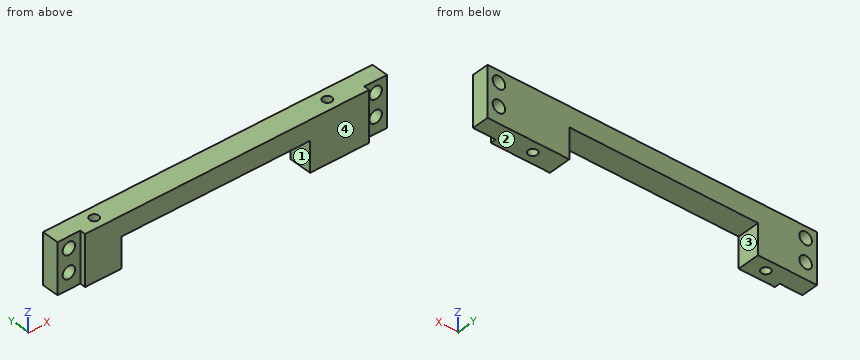
from build123d import *

# Parameters (mm, degrees)
MAIN_STOCK_START                         = 2.248090434
SKETCH_1_W                               = 57.95
SKETCH_1_H                               = 4
MAIN_STOCK_DEPTH                         = 8.851909566
SKETCH_2_W                               = 4
SKETCH_2_H                               = 1
CORNER_LEFT_RECTANGULAR_NOTCH_4X1_DEPTH  = 8.851909566
SKETCH_3_W                               = 4
SKETCH_3_H                               = 1
CORNER_RIGHT_RECTANGULAR_NOTCH_4X1_DEPTH = 8.851909566
SKETCH_4_R                               = 0.8
FRAME_2XD1P6_THROUGH_DEPTH               = 72.016485431
SKETCH_5_W                               = 33.203
SKETCH_5_H                               = 6.7
MERGED_INTERFACE_WINDOW_33P203X6P7_DEPTH = 4
SKETCH_6_R                               = 1.1
CORNER_REAR_4XD2P2_THROUGH_DEPTH         = 55.932071689


with BuildPart() as part:
    # 草图1 → Main_Stock (new body)
    with BuildSketch(Plane.XY.offset(MAIN_STOCK_START)):
        with Locations((24.675, 43.68)):
            Rectangle(SKETCH_1_W, SKETCH_1_H)
    extrude(amount=MAIN_STOCK_DEPTH)

    # 草图2 → Corner_Left_Rectangular_Notch_4x1 (cut)
    with BuildSketch(Plane.XY.offset(11.1)):
        with Locations((-2.3, 42.18)):
            Rectangle(SKETCH_2_W, SKETCH_2_H)
    extrude(amount=-CORNER_LEFT_RECTANGULAR_NOTCH_4X1_DEPTH, mode=Mode.SUBTRACT)

    # 草图3 → Corner_Right_Rectangular_Notch_4x1 (cut)
    with BuildSketch(Plane.XY.offset(11.1)):
        with Locations((51.65, 42.18)):
            Rectangle(SKETCH_3_W, SKETCH_3_H)
    extrude(amount=-CORNER_RIGHT_RECTANGULAR_NOTCH_4X1_DEPTH, mode=Mode.SUBTRACT)

    # 草图4 → Frame_2xD1p6_Through (cut, through all)
    with BuildSketch(Plane.XY.offset(11.1)):
        with Locations((3, 43.68)):
            Circle(SKETCH_4_R)
        with Locations((44, 43.68)):
            Circle(SKETCH_4_R)
    extrude(amount=-FRAME_2XD1P6_THROUGH_DEPTH, mode=Mode.SUBTRACT)

    # 草图5 → Merged_Interface_Window_33p203x6p7 (cut)
    with BuildSketch(Plane(origin=(0, 45.68, 0), x_dir=(1, 0, 0), z_dir=(0, 1, 0))):
        with Locations((22.6715, -4.25)):
            Rectangle(SKETCH_5_W, SKETCH_5_H)
    extrude(amount=-MERGED_INTERFACE_WINDOW_33P203X6P7_DEPTH, mode=Mode.SUBTRACT)

    # 草图6 → Corner_Rear_4xD2p2_Through (cut, through all)
    with BuildSketch(Plane(origin=(0, 45.68, 0), x_dir=(1, 0, 0), z_dir=(0, 1, 0))):
        with Locations(Location((-2.3, -5.1, 0), (0, 0, 270))):
            Circle(SKETCH_6_R)
        with Locations(Location((-2.3, -9.1, 0), (0, 0, 270))):
            Circle(SKETCH_6_R)
        with Locations(Location((51.65, -5.1, 0), (0, 0, 270))):
            Circle(SKETCH_6_R)
        with Locations(Location((51.65, -9.1, 0), (0, 0, 270))):
            Circle(SKETCH_6_R)
    extrude(amount=-CORNER_REAR_4XD2P2_THROUGH_DEPTH, mode=Mode.SUBTRACT)


solid = part.part
The model under review builds one solid part; all positions refer to its coordinate system, in mm. Face numbers are marked on the shaded views. A direction names the side the tool comes from. Coordinates: 2 decimals unless noted, no trailing zeros. Write each loop counter-clockwise with the first axis right and the second up, starting at its lowest first coordinate (ties: lowest second). Pieces come first, ordered by that corner, then holes. Notation, with made-up numbers: (25.25, 50.25) - (53.25, 50.25) arc R14 ccw to (53.25, 76.25) - close; hole circle Ø3 at (58, 67.5). An arc over 180 degrees is marked (long way). Answer as a JSON object with one key per item and string values. Group by question number.
1. Add section C-C (z = 9.1). Give the boundary of the cut face in (x, y), plus the area to 3 significant figures.
2. Mouldability with a two-part tool opening along X and no side actions: class the marked faces 3 and 4 as pulls with the +X half, pulls with the -X half, needs draft (parallel to the pull), parting line crosses it, or undercut.
3. Machinability: for the marked faces 1 and 2, which of the approach directions +Z, -Z, +X, -X, +Y, -Y give a long, thin tool a straight path to every point of the face, cutting with its end or side? Answer none if there is none.
4. Add section B-B (x = -2.3). Give the boundary of the cut face in (y, z).
5. Add section D-D (x = 44). Give the boundary of the cut face in (y, z).
6. Clearance check with flat-ended pins moving along their axes: pin 1 Ø1.3 at (x, z) = (-2.3, 9.1) entering from +Y; pin 2 Ø1.2 at (x, z) = (-1.5, 6) entering from -Y; pin 3 Ø2 at (x, y) = (23.5, 43.5) entering from -Z; pin 4 Ø1.1 at (y, z) = (42, 5) entering from -X. State where each tip first meets the part, or that it passes through.
7. Add section A-A (z = 5.1). Give the boundary of the cut face in (x, y).
8. To check wall thickness, follow probe 1 along X at (y, z) = (43.8, 2.5); probe 2 along X at (y, z) = (44.95, 9.1); probe 3 along X at (y, z) = (42.35, 6.25). State the ranges of each line that lie inside material, in increasing order.
Findings:
{
 "1": {"outline": "(-4.3, 42.68) - (-3.4, 42.68) - (-3.4, 45.68) - (-4.3, 45.68) - close; (-1.2, 42.68) - (-0.3, 42.68) - (-0.3, 41.68) - (49.65, 41.68) - (49.65, 42.68) - (50.55, 42.68) - (50.55, 45.68) - (-1.2, 45.68) - close; (52.75, 42.68) - (53.65, 42.68) - (53.65, 45.68) - (52.75, 45.68) - close; hole circle Ø1.6 at (3, 43.68); hole circle Ø1.6 at (44, 43.68)", "area": "207 mm²"},
 "2": {"face 3": "undercut", "face 4": "needs draft"},
 "3": {"face 1": "-Z, +Y, -Y", "face 2": "-Z, +X, -X, +Y, -Y"},
 "4": {"outline": "(42.68, 2.25) - (45.68, 2.25) - (45.68, 4) - (42.68, 4) - close; (42.68, 6.2) - (45.68, 6.2) - (45.68, 8) - (42.68, 8) - close; (42.68, 10.2) - (45.68, 10.2) - (45.68, 11.1) - (42.68, 11.1) - close"},
 "5": {"outline": "(41.68, 2.25) - (42.88, 2.25) - (42.88, 11.1) - (41.68, 11.1) - close; (44.48, 2.25) - (45.68, 2.25) - (45.68, 11.1) - (44.48, 11.1) - close"},
 "6": {"pin 1": "through", "pin 2": "y = 42.68", "pin 3": "z = 7.6", "pin 4": "x = -0.3"},
 "7": {"outline": "(-4.3, 42.68) - (-3.4, 42.68) - (-3.4, 45.68) - (-4.3, 45.68) - close; (-1.2, 42.68) - (-0.3, 42.68) - (-0.3, 41.68) - (6.07, 41.68) - (6.07, 45.68) - (-1.2, 45.68) - close; (39.27, 41.68) - (49.65, 41.68) - (49.65, 42.68) - (50.55, 42.68) - (50.55, 45.68) - (39.27, 45.68) - close; (52.75, 42.68) - (53.65, 42.68) - (53.65, 45.68) - (52.75, 45.68) - close; hole circle Ø1.6 at (3, 43.68); hole circle Ø1.6 at (44, 43.68)"},
 "8": {"probe 1": "-4.3 to 2.21, 3.79 to 6.07, 39.27 to 43.21, 44.79 to 53.65", "probe 2": "-4.3 to -3.4, -1.2 to 50.55, 52.75 to 53.65", "probe 3": "-0.3 to 6.07, 39.27 to 49.65"}
}
